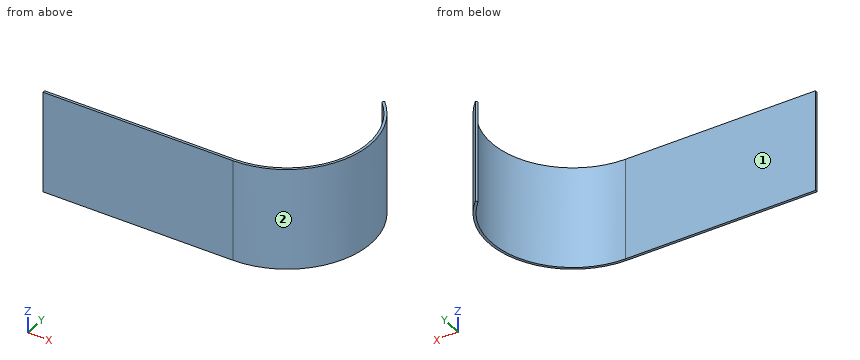
```python
from build123d import *

# Parameters (mm, degrees)
SURFACE_EXTRUDE1_1_DEPTH = 80
THICKEN1_T2              = 2


with BuildPart() as body_1:
    # Surface-Extrude1: a surface, the sketch's curves swept straight by 80 mm
    with BuildLine(Plane.XY, mode=Mode.PRIVATE) as surface_extrude1_1_path:
        Line((0, 0), (150, 0))
        ThreePointArc((150, 0), (209.531571016, 39.777724035), (195.563491861, 110))
    surface_extrude1_1 = Shell.extrude(surface_extrude1_1_path.wire(), (0 * SURFACE_EXTRUDE1_1_DEPTH, 0 * SURFACE_EXTRUDE1_1_DEPTH, 1 * SURFACE_EXTRUDE1_1_DEPTH))
    add(Solid.thicken(surface_extrude1_1, -THICKEN1_T2))


solid = body_1.part
```
The model under review builds one solid part; all positions refer to its coordinate system, in mm. Face numbers are marked on the shaded views. A direction names the side the tool comes from. Give positions to 0.01 mm unless a question says otherwise; leave off trailing zeros. Write each loop counter-clockwise with the first axis right and the second up, starting at its lowest first coordinate (ties: lowest second). Pieces come first, ordered by that corner, then holes.
(1) To check wall thickness, follow L1, parallel to Y at x = 12, z = 62; L2, parallel to X at y = 97.5, z = 43.5; L3, parallel to Y at x = 170, z = 67. State the ranges of each line that lie inside material, in increasing order.
(2) For P1, Ø1, axis at x = 44, z = 33.5, coming from the +Y side; P2, Ø5, axis at x = 181, z = 15, coming from the -Y side; P3, Ø5, axis at y = 50.5, z = 15.5, coming from the +X side, all flat-tipped, find the tip position at first contact; note any pin that passes through.
(3) Consider section A-A, the plane z = 41.5. Give the boundary of the cut face in (x, y).
(4) Consider section B-B, the plane x = 71.5. Give the boundary of the cut face in (y, z).
(5) Tool access review of the marked faces 1 and 2: name each direction out of +Z, -Z, +X, -X, +Y, -Y from which nothing blocks a thin tool from reaching the whole face with its end or side.
(6) Consider section C-C, the plane y = 8. Give the boundary of the cut face in (x, z), and give its area (3 significant figures).
Returned:
1. L1: y = -2 to 0
1. L2: x = 205.31 to 207.62
1. L3: y = 1.08 to 3.18
2. P1: stops at y = 0
2. P2: stops at y = 4.42
2. P3: stops at x = 215.44
3. outline: (0, -2) - (150, -2) arc R66.44 ccw to (196.98, 111.41) - (195.56, 110) arc R64.44 cw to (150, 0) - (0, 0) - close
4. outline: (-2, 0) - (0, 0) - (0, 80) - (-2, 80) - close
5. face 1: +Z, -Z, -X, +Y
5. face 2: +Z, -Z, +X
6. outline: (181.1, 0) - (185.05, 0) - (185.05, 80) - (181.1, 80) - close
6. area: 317 mm2
